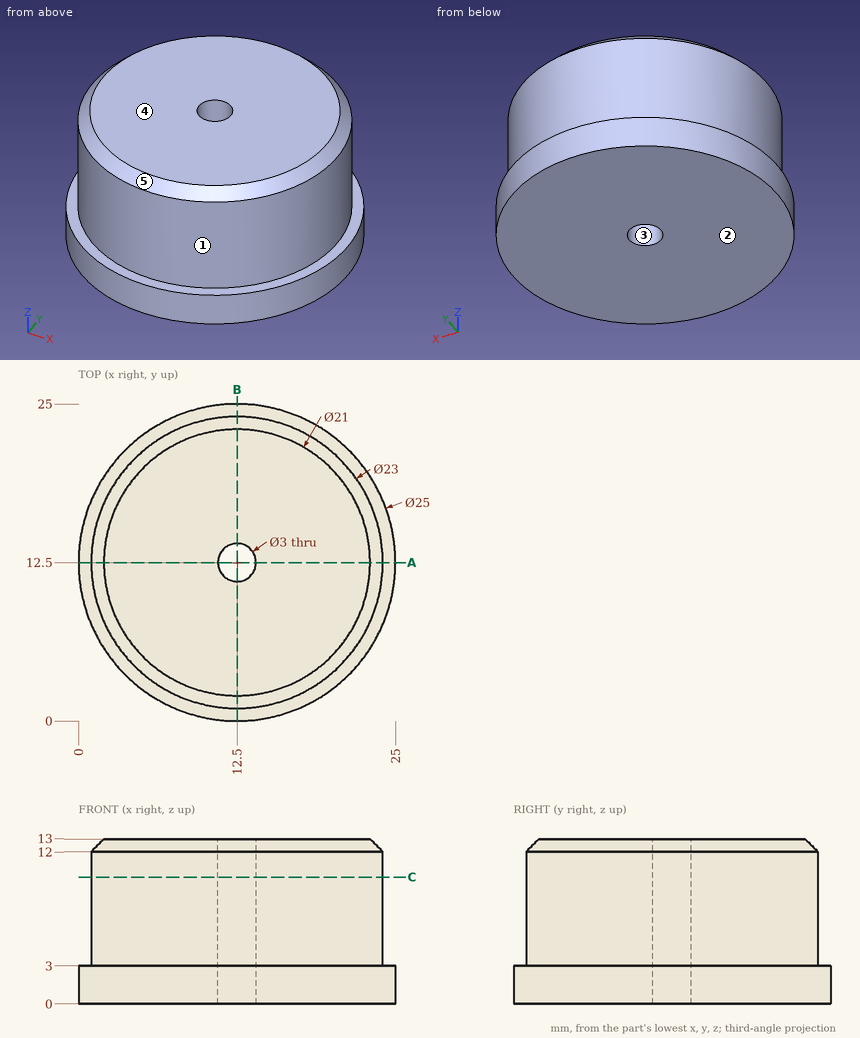
Check sheet for the drawn part. Datum: minimum x, y, z corner. Units: mm. A direction names the side the tool comes from. Round coordinates to 2 decimals unless told otherwise and drop trailing zeros. Loops run counter-clockwise (first coordinate to the right, second up) from the corner with the lowest first, then second, coordinate; pieces in that order, holes last.
Item 1: Cross-section at C-C on z = 10. Record the boundary of the cut face in (x, y).
Item 2: Access from +Z, -Z, +X, -X, +Y, -Y to the whole of each face (thin tool, end or side, straight path). Record for the marked faces 1 and 2.
Item 3: Cross-section at A-A on y = 12.5. Record the boundary of the cut face in (x, z), then the cut area to 3 significant figures.
Item 4: Gauge pin test, flat ends, axial feed: pin 1 (1 mm diameter, centred on y = 9, z = 9, fed in from +X); pin 2 (5 mm diameter, centred on x = 3, y = 3, fed in from +Z) (3 decimals); pin 3 (4 mm diameter, centred on x = 21.5, z = 5, fed in from +Y); pin 4 (12.5 mm diameter, centred on x = 13.5, y = 12, fed in from +Z). Record the tip position at first contact, or that the pin passes through.
Item 5: Thickness scan on line 1 (Y direction, x = 12.5, z = 4.5); line 2 (Y direction, x = 12.5, z = 2.75); line 3 (Z direction, x = 23, y = 7.5). Record the ranges inside material, lowest first.
Item 6: Mould release check, pull along X, two halves, no side actions. Record for the marked faces 3, 4 and 5: pulls with the +X half, pulls with the -X half, needs draft (parallel to the pull), parting line crosses it, or undercut.
Answer sheet:
1. outline: circle Ø23 at (12.5, 12.5); hole circle Ø3 at (12.5, 12.5)
2. face 1: +Z
2. face 2: -Z, +X, -X, +Y, -Y
3. outline: (0, 0) - (11, 0) - (11, 13) - (2, 13) - (1, 12) - (1, 3) - (0, 3) - close; (14, 0) - (25, 0) - (25, 3) - (24, 3) - (24, 12) - (23, 13) - (14, 13) - close
3. area: 265 mm2
4. pin 1: stops at x = 23.6
4. pin 2: stops at z = 12.565
4. pin 3: stops at y = 21.62
4. pin 4: stops at z = 13
5. line 1: y = 1 to 11, 14 to 24
5. line 2: y = 0 to 11, 14 to 25
5. line 3: z = 0 to 3
6. face 3: undercut
6. face 4: needs draft
6. face 5: parting line crosses it
